```python
from build123d import *

# Parameters (mm, degrees)
SKETCH1_R            = 30
BOSS_EXTRUDE1_DEPTH  = 20
CHAMFER1_SIZE        = 3
M3_CLEARANCE_HOLE1_D = 3.6


with BuildPart() as part:
    # Sketch1 → Boss-Extrude1 (new body)
    with BuildSketch(Plane(origin=(0, 0, 0), x_dir=(1, 0, 0), z_dir=(0, 1, 0))):
        with BuildLine():
            ThreePointArc((-54.559600438, 54.5), (-59.559600438, 0), (-54.559600438, -54.5))
            ThreePointArc((-54.559600438, -54.5), (-38.239092363, -66.232050808), (-19.918584287, -74.5))
            ThreePointArc((-19.918584287, -74.5), (29.779800219, -51.580127019), (74.478184725, -20))
            ThreePointArc((74.478184725, -20), (76.478184725, 0), (74.478184725, 20))
            ThreePointArc((74.478184725, 20), (29.779800219, 51.580127019), (-19.918584287, 74.5))
            ThreePointArc((-19.918584287, 74.5), (-38.239092363, 66.232050808), (-54.559600438, 54.5))
        make_face()
        Circle(SKETCH1_R, mode=Mode.SUBTRACT)
    extrude(amount=BOSS_EXTRUDE1_DEPTH)

    # Chamfer1
    chamfer1_edges = [part.edges().sort_by_distance(p)[0] for p in [
        (-38.239092363, 20, 66.232050808),
        (29.779800219, 20, 51.580127019),
        (-30, 20, 0),
        (76.478184725, 20, 0),
        (29.779800219, 20, -51.580127019),
        (-38.239092363, 20, -66.232050808),
        (-59.559600438, 20, 0),
    ]]
    chamfer(chamfer1_edges, length=CHAMFER1_SIZE)

    # M3 Clearance Hole1 (through all)
    with Locations(Plane(origin=(0, 20, 0), x_dir=(1, 0, 0), z_dir=(0, 1, 0))):
        with Locations((0, 0), (-43.145434031, 44.670326137), (-43.145434031, -44.670326137), (46.854565969, 0)):
            Hole(M3_CLEARANCE_HOLE1_D / 2)


solid = part.part
```
The listing builds one solid part. Answer for the finished solid, in the listing's coordinates (mm). Round coordinates to 2 decimals unless told otherwise and drop trailing zeros. Order: outer loops, then holes, each group sorted by start corner. A loop starts at its lowest first (then second) coordinate and runs counter-clockwise, first axis right, second up. Notation, with made-up numbers: (55.25, 2.25) - (66.25, 2.25) arc R9 ccw to (66.25, 17.25) - close; hole circle Ø10 at (63, 40). An arc over 180 degrees is marked (long way). Put each result on its own line as item: value. Start each with the question number.
(1) Find section B-B (y = 2). Give the vertices of the cut face in (x, z) (3 decimals), plus the area to 3 significant figures.
(2) Determine the mould class of faces 1 (the conical face through (29.35, 19.19, -49.3)), 2 (the cylindrical face through (-29.97, 8.38, -1.32)), 3 (the cylindrical face through (45.138, 9.86, -0.541)), 4 (the conical face through (-37.55, 18.85, 64.49)) for opening direction Z: released by +Z, released by -Z, zero draft, split by the parting line, or undercut.
(3) Find section A-A (z = 0). Give the vertices of the cut face in (x, y).
(4) Straight lines are drawn through the part: probe 1 along Z at (x, y) = (-19, 13.25); probe 2 along Z at (x, y) = (19, 15.25); probe 3 along X at (y, z) = (8.25, 23). For each, find the intervals that lie inside material, in ascending order. Write a range as from..to.
(5) Given P1, Ø3, axis at y = 16.5, z = -16.5, coming from the -X side; P2, Ø10, axis at y = 8, z = 35.5, coming from the +X side; P3, Ø2, axis at x = 4.5, y = 6, coming from the -Z side, each flat-ended and moving along its own axis, determine where each tip first touches the part or whether it passes through.
Reply:
1. outline: (-54.56, -54.5) arc R101 ccw to (-19.919, -74.5) arc R299.525 ccw to (74.478, -20) arc R101 ccw to (74.478, 20) arc R299.525 ccw to (-19.919, 74.5) arc R101 ccw to (-54.56, 54.5) arc R299.525 ccw to start; hole circle Ø3.6 at (-43.145, -44.67); hole circle Ø3.6 at (-43.145, 44.67); hole circle Ø60 at (0, 0); hole circle Ø3.6 at (46.855, 0)
1. area: 11,800 mm^2
2. face 1: released by -Z
2. face 2: undercut
2. face 3: undercut
2. face 4: released by +Z
3. outline: (-59.56, 0) - (-30, 0) - (-30, 17) - (-33, 20) - (-56.56, 20) - (-59.56, 17) - close; (30, 0) - (45.05, 0) - (45.05, 20) - (33, 20) - (30, 17) - close; (48.65, 0) - (76.48, 0) - (76.48, 17) - (73.48, 20) - (48.65, 20) - close
4. probe 1: -74.17..-23.22, 23.22..74.17
4. probe 2: -57.51..-23.22, 23.22..57.51
4. probe 3: -58.68..-19.26, 19.26..70.91
5. P1: x = -59.18
5. P2: x = 61.46
5. P3: z = -65.07
